Can you work these out from the model? Positions are in its coordinate system, mm. Coordinates: 2 decimals unless noted, no trailing zeros. Write each loop counter-clockwise with the first axis right and the second up, starting at its lowest first coordinate (ties: lowest second). Pieces come first, ordered by that corner, then holes. Notation, with made-up numbers: M 86,87 L 124,87 A15 ccw 124,108 Z; hole C 83,-17.75 d8. An arc over 180 degrees is marked long. Use one line per item in the form item = value. Start each with the question number.
Autodesk Inventor part; units mm, degrees
ref_plane "YZ Plane" through (0, 0, 0) normal (1, 0, 0) x (0, 1, 0)
ref_plane "XZ Plane" through (0, 0, 0) normal (0, 1, 0) x (-1, 0, 0)
ref_plane "XY Plane" through (0, 0, 0) normal (0, 0, 1) x (1, 0, 0)
sketch "Sketch1" plane through (0, 0, 0) normal (0, 0, 1) x (1, 0, 0)
  circle A0 centre (0, 0) radius 5.7
  dimension "d0" = 11.4
extrude "Extrusion1" add sketch "Sketch1" along normal blind 5
chamfer "Chamfer1" distance 0.8 angle 45 1 edges at (-5.7, 0, 5)
sketch "Sketch2" plane through (0, 0, 0) normal (0, 0, 1) x (1, 0, 0)
  circle A0 centre (0, 0) radius 2.9
  dimension "d6" = 5.8
extrude "Extrusion2" cut sketch "Sketch2" along normal blind 10
properties part number "Insert5mm"
1) Will this pin go through, and if not, where does the flat tip stop? pin 1 Ø1 at (x, z) = (3.5, 1) entering from +Y.
2) Please list where these lines run through material, in increasing order: line 1 (Y direction, x = 0, z = 1.5); line 2 (Y direction, x = -2.5, z = 1.5); line 3 (X direction, y = 1, z = 3.15).
3) If we mould it in two halves opening along Y, with no side actions, what happens to faces 1 (the face through (-0.1, -3.2, 5)), 2 (the face through (-4.5, 3.5, 2.1)), 3 (the face through (-2.9, -0.1, 2.5))? For each: +Y half, -Y half, draft (parallel to the pull), parting line (faces both ways), or undercut.
4) Suppose I cut it at D-D on z = 1.85. Please give me the cut outline in (x, y).
5) Suppose I cut it at A-A on y = 0. Please give me the cut outline in (x, z), and give its area (3 significant figures).
6) Suppose I cut it at C-C on z = 4.4. Please give me the cut outline in (x, y).
Computed values:
q1.pin_1 = 4.85
q2.line_1 = -5.7 to -2.9, 2.9 to 5.7
q2.line_2 = -5.12 to -1.47, 1.47 to 5.12
q2.line_3 = -5.61 to -2.72, 2.72 to 5.61
q3.face_1 = draft
q3.face_2 = parting line
q3.face_3 = undercut
q4.outline = C 0,0 d11.4; hole C 0,0 d5.8
q5.outline = M -5.7,0 L -2.9,0 L -2.9,5 L -4.9,5 L -5.7,4.2 Z; M 2.9,0 L 5.7,0 L 5.7,4.2 L 4.9,5 L 2.9,5 Z
q5.area = 27.4 mm²
q6.outline = C 0,0 d11; hole C 0,0 d5.8
